```python
from build123d import *

# Parameters (mm, degrees)
SKETCH_1_R          = 5
EXTRUDE_1_DEPTH     = 0.5
SKETCH_2_R          = 3.75
EXTRUDE_2_DEPTH     = 11
SKETCH_3_R          = 5
EXTRUDE_3_DEPTH     = 0.5
SKETCH_4_R          = 2.5
CUT_EXTRUDE_1_DEPTH = 14.928388277
FILLET_1_R          = 1


with BuildPart() as part:
    # 草图1 → 凸台-拉伸1 (new body)
    with BuildSketch(Plane.XY):
        Circle(SKETCH_1_R)
    extrude(amount=EXTRUDE_1_DEPTH)

    # 草图2 → 凸台-拉伸2 (add)
    with BuildSketch(Plane.XY.offset(0.5)):
        Circle(SKETCH_2_R)
    extrude(amount=EXTRUDE_2_DEPTH)

    # 草图3 → 凸台-拉伸3 (add)
    with BuildSketch(Plane.XY.offset(11.5)):
        Circle(SKETCH_3_R)
    extrude(amount=EXTRUDE_3_DEPTH)

    # 草图4 → 切除-拉伸1 (cut, through all)
    with BuildSketch(Plane.XY.offset(12)):
        Circle(SKETCH_4_R)
    extrude(amount=-CUT_EXTRUDE_1_DEPTH, mode=Mode.SUBTRACT)

    # 圆角1
    fillet_1_edges = [part.edges().sort_by_distance(p)[0] for p in [
        (-3.75, 0, 0.5),
        (-3.75, 0, 11.5),
    ]]
    fillet(fillet_1_edges, radius=FILLET_1_R)


solid = part.part
```
Geometry check sheet. Reference: the model listing, model coordinates, mm. Coordinates: 2 decimals unless noted, no trailing zeros. Write each loop counter-clockwise with the first axis right and the second up, starting at its lowest first coordinate (ties: lowest second). Pieces come first, ordered by that corner, then holes. Notation, with made-up numbers: M 48,8 L 92,8 A23 cw 92,27 Z; hole C 76.5,43.25 d9. An arc over 180 degrees is marked long. Use one line per item in the form item = value. Start each with the question number.
1) Section check D-D on z = 1. Enter the section's corners in (x, y).
2) Release check for a two-part mould opening along Y. For faces 1 (the flat face through (2, -2, 0)), 2 (the cylindrical face through (-3.746, 0.165, 5.937)), 3 (the cylindrical face through (-0.54, -2.44, 6.08)) record: pulls with the +Y half, pulls with the -Y half, needs draft (parallel to the pull), parting line crosses it, or undercut.
3) Go/stop test with flat-tipped pins: pin 1 Ø4 at (x, z) = (1, 2) entering from +Y; pin 2 Ø1.5 at (y, z) = (2, 6.5) entering from +X; pin 3 Ø6 at (y, z) = (-3.5, 5) entering from +X; pin 4 Ø2 at (x, z) = (-1, 5) entering from -Y. Record where each tip stops, or that it passes through.
4) Section check C-C on z = 10.25. Enter the section's corners in (x, y), and give its area (3 significant figures).
5) Section check A-A on y = 0. Enter the section's corners in (x, z), and give its area (3 significant figures).
6) Thickness scan on probe 1 along Y at (x, z) = (0, 7.5); probe 2 along Z at (x, y) = (2, -3.75); probe 3 along X at (y, z) = (-1.5, 9.25). Record the ranges inside material, lowest first. Write a range as from..to.
Responses:
q1.outline = C 0,0 d7.77; hole C 0,0 d5
q2.face_1 = needs draft
q2.face_2 = parting line crosses it
q2.face_3 = undercut
q3.pin_1 = 5
q3.pin_2 = 3.54
q3.pin_3 = 3.72
q3.pin_4 = -3.75
q4.outline = C 0,0 d7.5; hole C 0,0 d5
q4.area = 24.5 mm2
q5.outline = M -5,0 L -2.5,0 L -2.5,12 L -5,12 L -5,11.5 L -4.75,11.5 A1 cw -3.75,10.5 L -3.75,1.5 A1 cw -4.75,0.5 L -5,0.5 Z; M 2.5,0 L 5,0 L 5,0.5 L 4.75,0.5 A1 cw 3.75,1.5 L 3.75,10.5 A1 cw 4.75,11.5 L 5,11.5 L 5,12 L 2.5,12 Z
q5.area = 33.4 mm2
q6.probe_1 = -3.75..-2.5, 2.5..3.75
q6.probe_2 = 0..0.63, 11.37..12
q6.probe_3 = -3.44..-2, 2..3.44
